Read the model definition and answer for the solid it produces. Units are mm, in the model's axes. Coordinates: 2 decimals unless noted, no trailing zeros. Order: outer loops, then holes, each group sorted by start corner. A loop starts at its lowest first (then second) coordinate and runs counter-clockwise, first axis right, second up. Notation, with made-up numbers: (70, -5) -> (97, -5) arc R27 ccw to (97, 34) -> close; hole circle Ø2 at (4.5, 16.25). An arc over 180 degrees is marked (long way). Answer in a Markdown table with one row per item.
from build123d import *

# Parameters (mm, degrees)
EXTRUDE_1_DEPTH     = 6
SKETCH_2_R          = 6
SKETCH_2_R_2        = 4
EXTRUDE_2_DEPTH     = 12
SKETCH_3_R          = 2
CUT_EXTRUDE_1_DEPTH = 12
CHAMFER_1_SIZE      = 0.8
SKETCH_4_R          = 2
CUT_EXTRUDE_2_DEPTH = 6


with BuildPart() as part:
    # 草图1 → 凸台-拉伸1 (new body)
    with BuildSketch(Plane.XY):
        Polygon((6.92820323, 0), (3.464101615, 6), (-3.464101615, 6), (-6.92820323, 0), (-3.464101615, -6), (3.464101615, -6), align=None)
    extrude(amount=EXTRUDE_1_DEPTH)

    # 草图2 → 凸台-拉伸2 (add)
    with BuildSketch(Plane(origin=(0, 0, 0), x_dir=(-1, 0, 0), z_dir=(0, 0, -1))):
        with Locations(Location((0, 0, 0), (0, 0, 150))):
            Circle(SKETCH_2_R)
        Circle(SKETCH_2_R_2, mode=Mode.SUBTRACT)
    extrude(amount=EXTRUDE_2_DEPTH)

    # 草图3 → 切除-拉伸1 (cut)
    with BuildSketch(Plane.XY.offset(6)):
        Circle(SKETCH_3_R)
    extrude(amount=-CUT_EXTRUDE_1_DEPTH, mode=Mode.SUBTRACT)

    # 倒角1
    chamfer_1_edges = [part.edges().sort_by_distance(p)[0] for p in [
        (-2, 0, 6),
    ]]
    chamfer(chamfer_1_edges, length=CHAMFER_1_SIZE)

    # 草图4 → 切除-拉伸2 (cut, symmetric)
    with BuildSketch(Plane(origin=(0, 0, 0), x_dir=(1, 0, 0), z_dir=(0, 1, 0))):
        with Locations(Location((0, 7, 0), (0, 0, 270))):
            Circle(SKETCH_4_R)
    extrude(amount=CUT_EXTRUDE_2_DEPTH, both=True, mode=Mode.SUBTRACT)

    # 草图5 → 切除-旋转1 (revolve, cut)
    with BuildSketch(Plane(origin=(0, 0, 0), x_dir=(1, 0, 0), z_dir=(0, 1, 0))):
        Polygon((-6.92820323, 0), (-6.12820323, 0), (-6.92820323, -0.8), align=None)
        Polygon((-6.92820323, -5.2), (-6.92820323, -6), (-6.12820323, -6), align=None)
    revolve(axis=Axis((0, 0, 0), (0, 0, 1)), mode=Mode.SUBTRACT)


solid = part.part
Q1. The part is cut by section C-C (z = -1.75). Write down the section's boundary in (x, y), then the cut area to 3 significant figures.
Outcome:
| item | result |
|---|---|
| outline | circle Ø12 at (0, 0); hole circle Ø8 at (0, 0) |
| area | 62.8 mm² |
Q2. The part is cut by section B-B (z = -7). Write down the section's boundary in (x, y), then the cut area to 3 significant figures.
Outcome:
| item | result |
|---|---|
| outline | (-2, -5.66) -> (-2, -3.46) arc R4 cw to (-2, 3.46) -> (-2, 5.66) arc R6 ccw to start; (2, -5.66) arc R6 ccw to (2, 5.66) -> (2, 3.46) arc R4 cw to (2, -3.46) -> close |
| area | 46.3 mm² |
Q3. The part is cut by section A-A (z = 4). Write down the section's boundary in (x, y).
Outcome:
| item | result |
|---|---|
| outline | (-6.93, 0) -> (-3.46, -6) -> (3.46, -6) -> (6.93, 0) -> (3.46, 6) -> (-3.46, 6) -> close; hole circle Ø4 at (0, 0) |
Q4. For a pull along Y with two mould halves and no side action, classify faces 1 (the face through (0, -2, 3)), 2 (the face through (-5.22, -2.96, 2.96)), 3 (the face through (-6.36, 0.03, 5.77)) as pulls with the +Y half, pulls with the -Y half, needs draft (parallel to the pull), parting line crosses it, or undercut.
Outcome:
| item | result |
|---|---|
| face 1 | undercut |
| face 2 | pulls with the -Y half |
| face 3 | parting line crosses it |
Q5. Given pin 1 (2.5 mm diameter, centred on x = 0.5, y = -1, fed in from -Z); pin 2 (1 mm diameter, centred on y = -2, z = 0, fed in from +X); pin 3 (4.5 mm diameter, centred on x = 0, y = 0, fed in from +Z), each flat-ended and moving along its own axis, determine where each tip first touches the part or whether it passes through.
Outcome:
| item | result |
|---|---|
| pin 1 | z = 0 |
| pin 2 | x = 6.05 |
| pin 3 | z = 5.45 |
Q6. Consider line 1 (Z direction, x = 0, y = 4.8); line 2 (Y direction, x = 0, z = 3.6); line 3 (Y direction, x = -1.5, z = -2.25). Determine where each line is inside the solid, lowest interval first.
Outcome:
| item | result |
|---|---|
| line 1 | -12 to -9, -5 to 6 |
| line 2 | -6 to -2, 2 to 6 |
| line 3 | -5.81 to -3.71, 3.71 to 5.81 |
